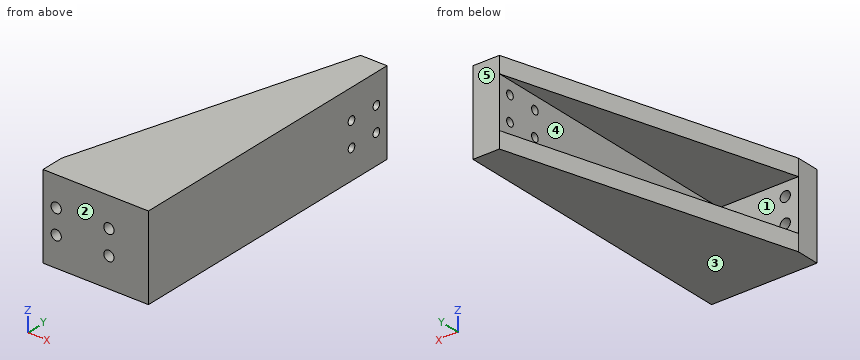
```python
from build123d import *

# Parameters (mm, degrees)
BOSS_EXTRUDE1_DEPTH = 25.4
RIB1_REACH          = 100.839
SKETCH4_WALL_W      = 286.07835369
SKETCH4_WALL_H      = 5
CUT_EXTRUDE2_REACH  = 94.51
SKETCH5_R           = 1.55
M3_TAPPED_HOLE2_D   = 2.5


with BuildPart() as part:
    # Sketch1 → Boss-Extrude1 (new body)
    with BuildSketch(Plane.XY):
        Polygon((0, 0), (0, 7), (24, 7), (24, 90), (32, 90), (32, 0), align=None)
    extrude(amount=BOSS_EXTRUDE1_DEPTH)

    # Sketch4 wall → Rib1 (add, up to next)
    with BuildSketch(Plane(origin=(12, 48.5, 25.4), x_dir=(-0.277777033563, -0.960645574406, 0), z_dir=(0.960645574406, -0.277777033563, 0)), mode=Mode.PRIVATE) as rib1_sk1:
        with Locations((0, 2.5)):
            Rectangle(SKETCH4_WALL_W, SKETCH4_WALL_H)
    rib1_tool1 = extrude(rib1_sk1.sketch, amount=RIB1_REACH, mode=Mode.PRIVATE) - part.part
    rib1 = rib1_tool1.solids().sort_by_distance((12, 48.5, 25.4))[0]
    add(rib1)

    # Mirror1: Rib1 across plane
    add(rib1.mirror(Plane.XY.offset(12.7)))

    # Sketch5 → Cut-Extrude2 (cut, up to next)
    with BuildSketch(Plane(origin=(0, 7, 0), x_dir=(1, 0, 0), z_dir=(0, 1, 0)), mode=Mode.PRIVATE) as cut_extrude2_sk1:
        with Locations(Location((4, -9, 0), (0, 0, 270))):
            Circle(SKETCH5_R)
    cut_extrude2_tool1 = extrude(cut_extrude2_sk1.sketch, amount=-CUT_EXTRUDE2_REACH, mode=Mode.PRIVATE) & part.part
    # Sketch5 → Cut-Extrude2 (cut, up to next)
    with BuildSketch(Plane(origin=(0, 7, 0), x_dir=(1, 0, 0), z_dir=(0, 1, 0)), mode=Mode.PRIVATE) as cut_extrude2_sk2:
        with Locations(Location((20, -9, 0), (0, 0, 270))):
            Circle(SKETCH5_R)
    cut_extrude2_tool2 = extrude(cut_extrude2_sk2.sketch, amount=-CUT_EXTRUDE2_REACH, mode=Mode.PRIVATE) & part.part
    # Sketch5 → Cut-Extrude2 (cut, up to next)
    with BuildSketch(Plane(origin=(0, 7, 0), x_dir=(1, 0, 0), z_dir=(0, 1, 0)), mode=Mode.PRIVATE) as cut_extrude2_sk3:
        with Locations(Location((20, -16.4, 0), (0, 0, 270))):
            Circle(SKETCH5_R)
    cut_extrude2_tool3 = extrude(cut_extrude2_sk3.sketch, amount=-CUT_EXTRUDE2_REACH, mode=Mode.PRIVATE) & part.part
    # Sketch5 → Cut-Extrude2 (cut, up to next)
    with BuildSketch(Plane(origin=(0, 7, 0), x_dir=(1, 0, 0), z_dir=(0, 1, 0)), mode=Mode.PRIVATE) as cut_extrude2_sk4:
        with Locations(Location((4, -16.4, 0), (0, 0, 270))):
            Circle(SKETCH5_R)
    cut_extrude2_tool4 = extrude(cut_extrude2_sk4.sketch, amount=-CUT_EXTRUDE2_REACH, mode=Mode.PRIVATE) & part.part
    add(cut_extrude2_tool1.solids().sort_by_distance((4, 7, 9))[0], mode=Mode.SUBTRACT)
    add(cut_extrude2_tool2.solids().sort_by_distance((20, 7, 9))[0], mode=Mode.SUBTRACT)
    add(cut_extrude2_tool3.solids().sort_by_distance((20, 7, 16.4))[0], mode=Mode.SUBTRACT)
    add(cut_extrude2_tool4.solids().sort_by_distance((4, 7, 16.4))[0], mode=Mode.SUBTRACT)

    # M3 Tapped Hole2 (through all)
    with Locations(Plane(origin=(32, 0, 0), x_dir=(0, 0, -1), z_dir=(1, 0, 0))):
        with Locations((-9, 86), (-16.4, 76.6), (-16.4, 86), (-9, 76.6)):
            Hole(M3_TAPPED_HOLE2_D / 2)


solid = part.part
```
Part model, mm, in its own coordinate system. Face numbers are marked on the shaded views. A direction names the side the tool comes from. Give positions to 0.01 mm unless a question says otherwise; leave off trailing zeros. Loops run counter-clockwise (first coordinate to the right, second up) from the corner with the lowest first, then second, coordinate; pieces in that order, holes last. Notation, with made-up numbers: M 41,64.25 L 71,64.25 A24 ccw 71,83.25 Z; hole C 32.25,58 d4. An arc over 180 degrees is marked long. Return JSON: item names as keys, results as strings.
1) Drill centre lines: line 1 (Y direction, x = 28.75, z = 9); line 2 (X direction, y = 2, z = 16.4); line 3 (Z direction, x = 11.5, y = 46.5). Where is each one in solid material? Low to high.
Calculated:
{"line 1": "y = 0 to 75.35, 77.85 to 84.75, 87.25 to 90", "line 2": "x = 0 to 2.45, 5.55 to 18.45, 21.55 to 32", "line 3": "z = 0 to 5, 20.4 to 25.4"}
2) Saw through at D-D, the plane y = 76.6. List the corners of the cut face in (x, z).
Calculated:
{"outline": "M 20.13,0 L 32,0 L 32,7.75 L 24,7.75 L 24,5 L 20.13,5 Z; M 20.13,20.4 L 24,20.4 L 24,17.65 L 32,17.65 L 32,25.4 L 20.13,25.4 Z; M 24,10.25 L 32,10.25 L 32,15.15 L 24,15.15 Z"}
3) Flat gauge pins, fed straight in: pin 1 Ø3 at (y, z) = (78, 14.5) entering from -X; pin 2 Ø1.9 at (x, z) = (4, 9) entering from +Y; pin 3 Ø6 at (x, z) = (15, 10) entering from +Y. Where does each tip first touch, or does it go through?
Calculated:
{"pin 1": "stops at x = 24", "pin 2": "passes through", "pin 3": "stops at y = 7"}
4) Saw through at C-C, the plane x = 4. List the corners of the cut face in (y, z).
Calculated:
{"outline": "M 0,0 L 20.83,0 L 20.83,5 L 7,5 L 7,7.45 L 0,7.45 Z; M 0,10.55 L 7,10.55 L 7,14.85 L 0,14.85 Z; M 0,17.95 L 7,17.95 L 7,20.4 L 20.83,20.4 L 20.83,25.4 L 0,25.4 Z"}
5) 3-axis set-ups, long thin cutter, end or side, ignore diameter. For the marked faces 4 and 5: which of +Z, -Z, +X, -X, +Y, -Y reach the whole face in a straight line?
Calculated:
{"face 4": "-X, +Y", "face 5": "+Z, -Z, +X, -X, +Y"}
6) Pull direction Z, two halves, no side cores. Call the marked faces 1, 2 and 3: released by +Z, released by -Z, zero draft, split by the parting line, or undercut.
Calculated:
{"face 1": "undercut", "face 2": "zero draft", "face 3": "released by -Z"}
7) Saw through at A-A, the plane z = 16.4. List the corners of the cut face in (x, y), then the cut area to 3 significant figures.
Calculated:
{"outline": "M 0,0 L 2.45,0 L 2.45,7 L 0,7 Z; M 5.55,0 L 18.45,0 L 18.45,7 L 5.55,7 Z; M 21.55,0 L 32,0 L 32,75.35 L 24,75.35 L 24,7 L 21.55,7 Z; M 24,77.85 L 32,77.85 L 32,84.75 L 24,84.75 Z; M 24,87.25 L 32,87.25 L 32,90 L 24,90 Z", "area": "805 mm2"}
8) Saw through at B-B, the plane y = 48.5. List the corners of the cut face in (x, z).
Calculated:
{"outline": "M 12,0 L 32,0 L 32,25.4 L 12,25.4 L 12,20.4 L 24,20.4 L 24,5 L 12,5 Z"}
